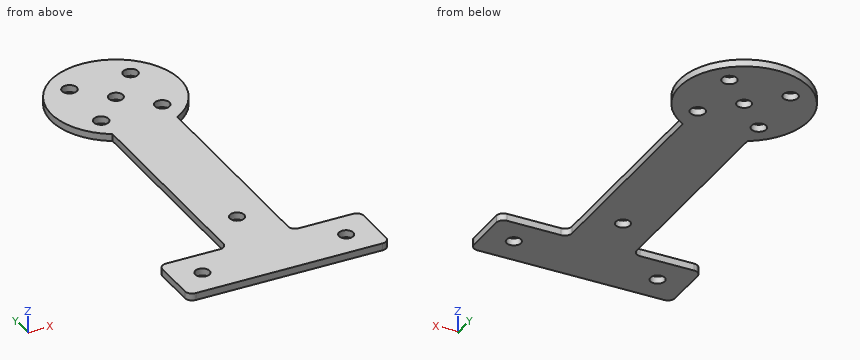
```python
from build123d import *

# Parameters (mm, degrees)
SKETCH_1_R      = 2
SKETCH_1_R_2    = 2.05
EXTRUDE_1_DEPTH = 2
FILLET_1_R      = 2


with BuildPart() as part:
    # 草图1 → 凸台-拉伸1 (new body)
    with BuildSketch(Plane.XY):
        with BuildLine():
            Line((14.659550972, 19.565520938), (14.659550972, 35.565520938))
            Line((14.659550972, 35.565520938), (-4.340449028, 35.565520938))
            Line((-4.340449028, 35.565520938), (-4.340449028, 96.97706367))
            ThreePointArc((-4.340449028, 96.97706367), (-13.340449028, 130.565520938), (-22.340449028, 96.97706367))
            Line((-22.340449028, 96.97706367), (-22.340449028, 35.565520938))
            Line((-22.340449028, 35.565520938), (-41.340449028, 35.565520938))
            Line((-41.340449028, 35.565520938), (-41.340449028, 19.565520938))
            Line((-41.340449028, 19.565520938), (14.659550972, 19.565520938))
        make_face()
        with Locations((-33.340449028, 27.565520938)):
            Circle(SKETCH_1_R, mode=Mode.SUBTRACT)
        with Locations(Location((6.659550972, 27.565520938, 0), (0, 0, 180))):
            Circle(SKETCH_1_R, mode=Mode.SUBTRACT)
        with Locations((-13.340449028, 112.565520938)):
            Circle(SKETCH_1_R, mode=Mode.SUBTRACT)
        with Locations((-13.340449028, 47.565520938)):
            Circle(SKETCH_1_R, mode=Mode.SUBTRACT)
        with Locations((-4.840449028, 121.065520938)):
            Circle(SKETCH_1_R_2, mode=Mode.SUBTRACT)
        with Locations((-4.840449028, 104.065520938)):
            Circle(SKETCH_1_R_2, mode=Mode.SUBTRACT)
        with Locations((-21.840449028, 104.065520938)):
            Circle(SKETCH_1_R_2, mode=Mode.SUBTRACT)
        with Locations((-21.840449028, 121.065520938)):
            Circle(SKETCH_1_R_2, mode=Mode.SUBTRACT)
    extrude(amount=EXTRUDE_1_DEPTH)

    # 圆角1
    fillet_1_edges = [part.edges().sort_by_distance(p)[0] for p in [
        (-41.340449028, 19.565520938, 1),
        (-41.340449028, 35.565520938, 1),
        (-22.340449028, 35.565520938, 1),
        (-4.340449028, 35.565520938, 1),
        (14.659550972, 35.565520938, 1),
        (14.659550972, 19.565520938, 1),
    ]]
    fillet(fillet_1_edges, radius=FILLET_1_R)


solid = part.part
```
The listing builds one solid part. Answer for the finished solid, in the listing's coordinates (mm). Give positions to 0.01 mm unless a question says otherwise; leave off trailing zeros. Order: outer loops, then holes, each group sorted by start corner. A loop starts at its lowest first (then second) coordinate and runs counter-clockwise, first axis right, second up. Notation, with made-up numbers: (-5, 30.25) -> (27, 30.25) arc R22 cw to (27, 54.25) -> close; hole circle Ø2 at (-15, 5.25). An arc over 180 degrees is marked (long way). One line per item, written item: value.
1) Find section A-A, the plane x = -27.5. Determine the outline of the cut face in (y, z).
Reported:
outline: (19.57, 0) -> (35.57, 0) -> (35.57, 2) -> (19.57, 2) -> close; (101.45, 0) -> (123.68, 0) -> (123.68, 2) -> (101.45, 2) -> close
2) Find the intervals of material crossed by line 1 (Y direction, x = -13.5, z = 0.8); line 2 (Y direction, x = -14, z = 0.2); line 3 (Y direction, x = -23.5, z = 0.8), in increasing order.
Reported:
line 1: y = 19.57 to 45.57, 49.56 to 110.57, 114.56 to 130.56
line 2: y = 19.57 to 45.68, 49.45 to 110.68, 114.45 to 130.55
line 3: y = 19.57 to 35.75, 97.71 to 102.86, 105.27 to 119.86, 122.27 to 127.42
3) Find section C-C, the plane y = 70.5. Determine the outline of the cut face in (x, z).
Reported:
outline: (-22.34, 0) -> (-4.34, 0) -> (-4.34, 2) -> (-22.34, 2) -> close
4) A flat-ended cylindrical pin translates along its axis: P1, Ø3.5, axis at x = -4.84, y = 104.07, coming from the +Z side. Find the tip coordinate at first contact, or state that the pin passes through.
Reported:
P1: passes through
5) Find section B-B, the plane z = 0.65. Count the separate pieces of the cut face and the enclosed holes in it, plus the area to 3 significant figures.
Reported:
separate pieces: 1
enclosed holes: 8
area: 2,890 mm^2
